Input: dimensioned drawing with shaded views. Units: mm. Origin: part minimum x, y, z. A direction names the side the tool comes from. Give positions to 0.01 mm unless a question says otherwise; leave off trailing zeros. Order: outer loops, then holes, each group sorted by start corner. A loop starts at its lowest first (then second) coordinate and runs counter-clockwise, first axis right, second up. Notation, with made-up numbers: M 6,0 L 31,0 A13 cw 31,25 Z; hole C 38.25,11.5 d5. An arc over 180 degrees is marked long. Answer in a Markdown table with one row per item. Add a question column.
(1) Section query D-D, the plane y = 17.5. Return loops of the section in (x, z), plus the area to 3 significant figures.
(2) Pin query (flat end, axial travel): P1, Ø1.1, axis at x = 0.5, z = 2, coming from the -Y side; P2, Ø0.8, axis at y = 27.5, z = 3, coming from the -X side; P3, Ø1.1, axis at x = 3.5, z = 1, coming from the +Y side; P4, Ø8, axis at x = 5.5, y = 9.5, coming from the -Z side. Return the tip coordinate at first contact, or that it passes through.
(3) Section query C-C, the plane x = 2.5. Return loops of the section in (y, z).
(4) Set-up query: the marked faces 5, 6, 7, 8 and 9. Return all of +Z, -Z, +X, -X, +Y, -Y with unobstructed straight access to the full face (end or side cutting, diameter ignored); none if empty.
(5) Mould query, pull axis Y, two halves, no side actions, for the marked faces 1, 2, 3 and 4. Classes: pulls with the +Y half, pulls with the -Y half, needs draft (parallel to the pull), parting line crosses it, or undercut.
(6) Section query B-B, the plane y = 14. Return loops of the section in (x, z).
(7) Material intervals for line 1 along Y through (x, z) = (17, 2.35); line 2 along Z through (x, y) = (1.3, 14); line 3 along X through (y, z) = (7.5, 3.4), sorted ascending.
(8) Section query A-A, the plane x = 22.25. Return loops of the section in (y, z).
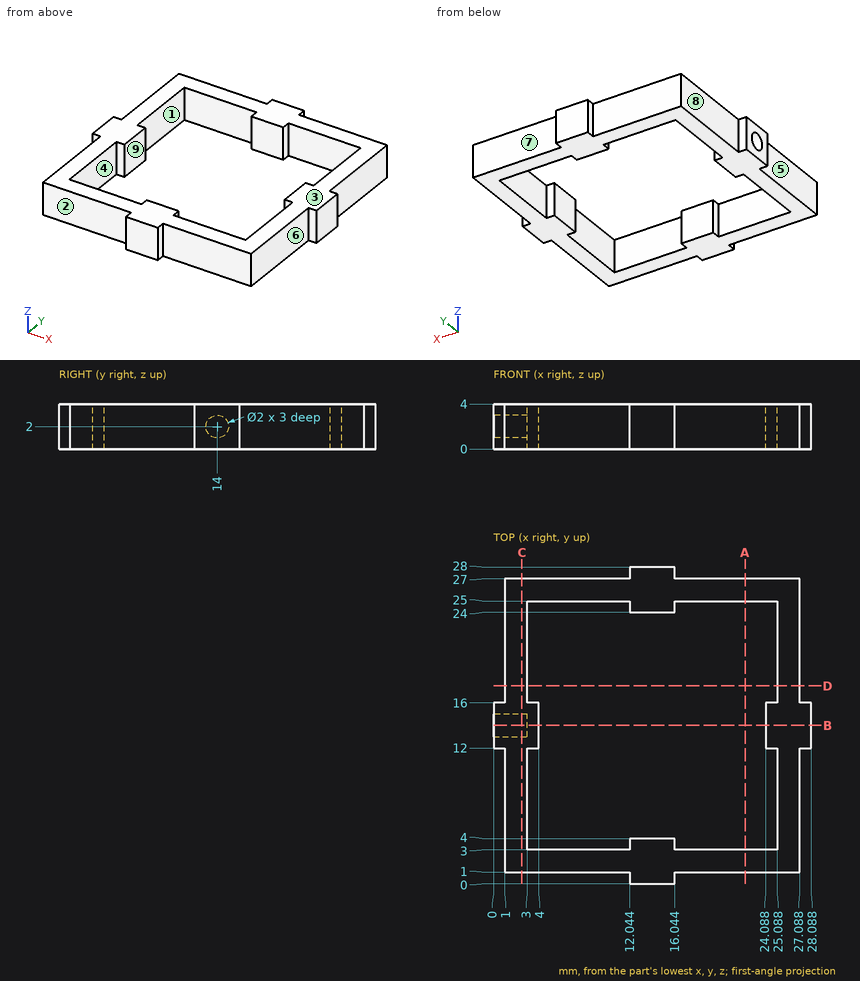
Values follow:
| question | item | result |
|---|---|---|
| 1 | outline | M 1,0 L 3,0 L 3,4 L 1,4 Z; M 25.09,0 L 27.09,0 L 27.09,4 L 25.09,4 Z |
| 1 | area | 16.0 mm² |
| 2 | P1 | stops at y = 1 |
| 2 | P2 | stops at x = 12.04 |
| 2 | P3 | stops at y = 27 |
| 2 | P4 | stops at z = 0 |
| 3 | outline | M 1,0 L 27,0 L 27,4 L 1,4 Z; hole C 14,2 d2 |
| 4 | face 5 | +Z, -Z, -X, -Y |
| 4 | face 6 | +Z, -Z, +X, -Y |
| 4 | face 7 | +Z, -Z, +X, +Y |
| 4 | face 8 | +Z, -Z, -X, +Y |
| 4 | face 9 | +Z, -Z |
| 5 | face 1 | undercut |
| 5 | face 2 | pulls with the -Y half |
| 5 | face 3 | needs draft |
| 5 | face 4 | undercut |
| 6 | outline | M 0,0 L 4,0 L 4,4 L 0,4 L 0,3 L 3,3 L 3,1 L 0,1 Z; M 24.09,0 L 28.09,0 L 28.09,4 L 24.09,4 Z |
| 7 | line 1 | y = 1 to 3, 25 to 27 |
| 7 | line 2 | z = 0 to 1, 3 to 4 |
| 7 | line 3 | x = 1 to 3, 25.09 to 27.09 |
| 8 | outline | M 1,0 L 3,0 L 3,4 L 1,4 Z; M 25,0 L 27,0 L 27,4 L 25,4 Z |
